The drawing under review shows one solid part. Ordinate dimensions are in mm from its lowest x, y, z. Coordinates: 2 decimals unless noted, no trailing zeros. Return JSON: item names as keys, results as strings.
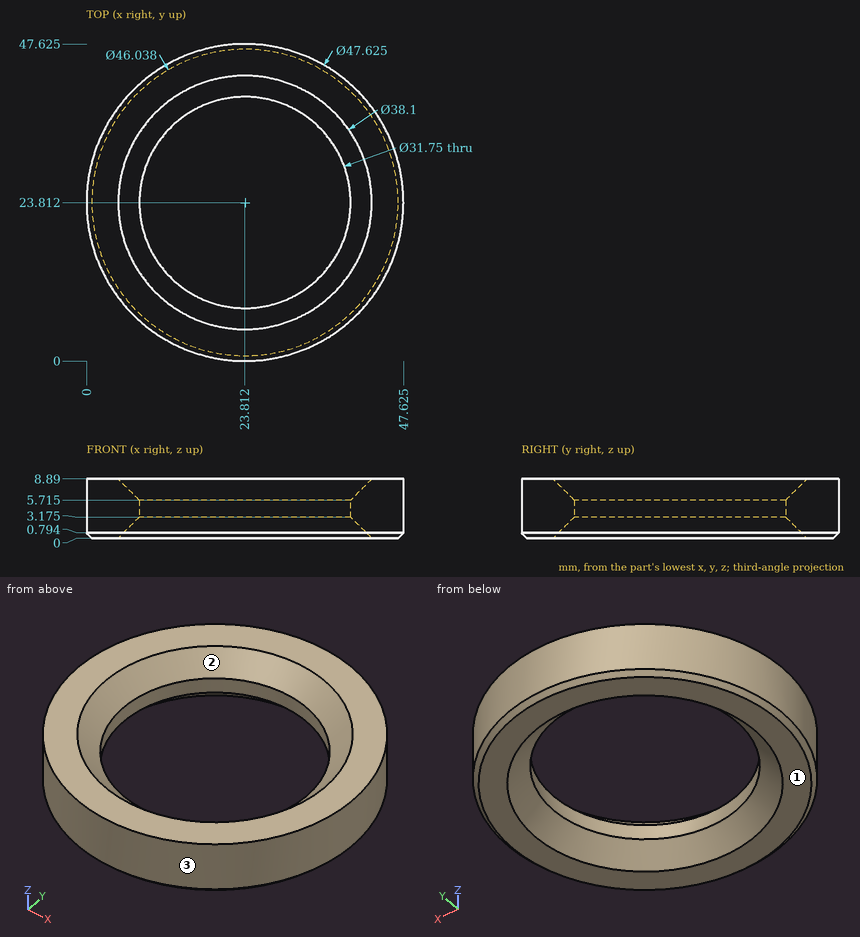
1. To check wall thickness, follow line 1 (Y direction, x = 20, z = 8.25) (1 decimal); line 2 (X direction, y = 26.5, z = 4); line 3 (Y direction, x = 35, z = 7.75) (1 decimal). State the ranges of each line that lie inside material, in increasing order.
Check values:
{"line 1": "0.3 to 5.8, 41.8 to 47.3", "line 2": "0.15 to 8.17, 39.46 to 47.47", "line 3": "2.8 to 9.8, 37.8 to 44.8"}
2. Insertion check: pin 1 Ø3 at (x, y) = (28.5, 40.5) entering from +Z (1 decimal); pin 2 Ø3 at (x, z) = (7, 5.5) entering from -Y (1 decimal); pin 3 Ø1.5 at (x, z) = (12.5, 1.5) entering from +Y (1 decimal). Each pin has a flat end and moves straight along its axis. Give the tip position at first contact, or say it passes through.
Check values:
{"pin 1": "z = 8.7", "pin 2": "y = 5.6", "pin 3": "y = 45.2"}
3. The part is to be moulded in two halves that separate along X. For the marked faces 1, 2 and 3, say which applies: released by +X, released by -X, zero draft, split by the parting line, or undercut.
Check values:
{"face 1": "zero draft", "face 2": "undercut", "face 3": "split by the parting line"}
